```python
from build123d import *

# Parameters (mm, degrees)
F0_W     = 200
F0_H     = 100
F1_DEPTH = 5
F2_W     = 50
F2_H     = 50
F3_DEPTH = 10
F4_W     = 40
F4_H     = 40
F5_DEPTH = 10
F6_W     = 10
F6_H     = 10
F7_DEPTH = 20


with BuildPart() as f1:
    # F0 (on Top) → F1 (new body)
    with BuildSketch(Plane.XY):
        with Locations((0, 1.493815)):
            Rectangle(F0_W, F0_H)
    extrude(amount=F1_DEPTH)

    # F2 (on face) → F3 (join)
    with BuildSketch(Plane.XY.offset(5)):
        Rectangle(F2_W, F2_H)
    extrude(amount=F3_DEPTH)

    # F4 (on face) → F5 (cut)
    with BuildSketch(Plane.XY.offset(15)):
        Rectangle(F4_W, F4_H)
    extrude(amount=-F5_DEPTH, mode=Mode.SUBTRACT)

    # F6 (on face) → F7 (join)
    with BuildSketch(Plane.XY.offset(5)):
        Rectangle(F6_W, F6_H)
    extrude(amount=F7_DEPTH)


solid = f1.part
```
Read the model definition and answer for the solid it produces. Units are mm, in the model's axes. A direction names the side the tool comes from. Give positions to 0.01 mm unless a question says otherwise; leave off trailing zeros. Loops run counter-clockwise (first coordinate to the right, second up) from the corner with the lowest first, then second, coordinate; pieces in that order, holes last.
Item 1: Each of these flat-tipped pins is pushed along its axis until it touches: pin 1 Ø11 at (y, z) = (2, 8.5) entering from +X; pin 2 Ø11 at (x, z) = (7, 12) entering from +Y; pin 3 Ø5 at (y, z) = (1.5, 19) entering from +X; pin 4 Ø3 at (x, z) = (-9, 12) entering from -Y. Where does it stop, or does it pass through?
Item 2: Find the intervals of material crossed by line 1 along Y through (x, z) = (4.5, 10.5); line 2 along Z through (x, y) = (-7.5, 9); line 3 along X through (y, z) = (1, 19.5), in increasing order.
Item 3: The part is cut by section C-C (x = 73.5). Write down the section's boundary in (y, z), and give its area (3 significant figures).
Item 4: The part is cut by section D-D (z = 19.5). Write down the section's boundary in (x, y), and give its area (3 significant figures).
Item 5: The part is cut by section B-B (y = -12). Write down the section's boundary in (x, z), and give its area (3 significant figures).
Item 6: The mould has two halves that part along X. Classify faces 4 (the flat face through (-5, 0, 15)), 5 (the flat face through (100, 1, 2)), 6 (the flat face through (-1, 36, 5)): released by +X, released by -X, zero draft, split by the parting line, or undercut.
Item 7: The part is cut by section A-A (z = 8.5). Write down the section's boundary in (x, y).
Item 8: For faces 1 (the flat face through (5, 0, 15)), 2 (the flat face through (0, 25, 10)), 3 (the flat face through (25, 0, 10)), determine the directions among +Z, -Z, +X, -X, +Y, -Y from which every point of the face is accessible in a straight line to the end or side of a thin tool.
Taken from the geometry:
1. pin 1: stops at x = 100
1. pin 2: stops at y = 25
1. pin 3: stops at x = 5
1. pin 4: stops at y = -25
2. line 1: y = -25 to -20, -5 to 5, 20 to 25
2. line 2: z = 0 to 5
2. line 3: x = -5 to 5
3. outline: (-48.51, 0) - (51.49, 0) - (51.49, 5) - (-48.51, 5) - close
3. area: 500 mm2
4. outline: (-5, -5) - (5, -5) - (5, 5) - (-5, 5) - close
4. area: 100 mm2
5. outline: (-100, 0) - (100, 0) - (100, 5) - (25, 5) - (25, 15) - (20, 15) - (20, 5) - (-20, 5) - (-20, 15) - (-25, 15) - (-25, 5) - (-100, 5) - close
5. area: 1,100 mm2
6. face 4: undercut
6. face 5: released by +X
6. face 6: zero draft
7. outline: (-25, -25) - (25, -25) - (25, 25) - (-25, 25) - close; (-5, -5) - (5, -5) - (5, 5) - (-5, 5) - close; hole (-20, -20) - (20, -20) - (20, 20) - (-20, 20) - close
8. face 1: +Z
8. face 2: +Z, +X, -X, +Y
8. face 3: +Z, +X, +Y, -Y
